Model file for the job. Use its own axes, mm. Round coordinates to 2 decimals unless told otherwise and drop trailing zeros. Loops run counter-clockwise (first coordinate to the right, second up) from the corner with the lowest first, then second, coordinate; pieces in that order, holes last. Notation, with made-up numbers: M 80,-35.5 L 130,-35.5 A19 ccw 130,-30.5 Z; hole C -31,-1 d11. An arc over 180 degrees is marked long. Use a Markdown table: item, result. Add a question column.
Q1. Cut at D-D (x = -63.5). Give the cut face in (y, z).
Q2. Cut at B-B (z = 0). Give the cut face in (x, y).
Q3. Cut at A-A (x = 40.5). Give the cut face in (y, z), plus the area to 3 significant figures.
Q4. Probe line 1 (X direction, y = 1.3, z = 0); line 2 (X direction, y = -1.15, z = -9.5); line 3 (Z direction, x = -63.5, y = -0.45). List the from-to ranges inside material, lowest first. Write a range as from..to.
Q5. Pin check, flat tip, straight feed: pin 1 (2.5 mm diameter, centred on x = -63.5, z = 0, fed in from -Y). Stop position of the tip, or through.
Q6. Cut at C-C (y = 0.15). State how many separate pieces and enclosed holes the cut face has, plus the area to 3 significant figures.
from build123d import *

# Parameters (mm, degrees)
SKETCH1_W           = 152.4
SKETCH1_H           = 63.5
SKETCH1_R           = 1.4605
SKETCH1_W_2         = 16.002
SKETCH1_H_2         = 28.702
BOSS_EXTRUDE1_DEPTH = 2.667
FILLET1_R           = 1.27
FILLET2_R           = 6.35


with BuildPart() as part:
    # Sketch1 → Boss-Extrude1 (new, symmetric)
    with BuildSketch(Plane(origin=(0, 0, 0), x_dir=(1, 0, 0), z_dir=(0, 1, 0))):
        Rectangle(SKETCH1_W, SKETCH1_H)
        with Locations(Location((63.5, 0, 0), (0, 0, 270))):
            Circle(SKETCH1_R, mode=Mode.SUBTRACT)
        with Locations(Location((-63.5, 0, 0), (0, 0, 90))):
            Circle(SKETCH1_R, mode=Mode.SUBTRACT)
        with Locations((-38.1, 0)):
            Rectangle(SKETCH1_W_2, SKETCH1_H_2, mode=Mode.SUBTRACT)
        Rectangle(SKETCH1_W_2, SKETCH1_H_2, mode=Mode.SUBTRACT)
        with Locations((38.1, 0)):
            Rectangle(SKETCH1_W_2, SKETCH1_H_2, mode=Mode.SUBTRACT)
    extrude(amount=BOSS_EXTRUDE1_DEPTH, both=True)

    # Fillet1
    fillet1_edges = [part.edges().sort_by_distance(p)[0] for p in [
        (-30.099, 0, 14.351),
        (-30.099, 0, -14.351),
        (-46.101, 0, -14.351),
        (-46.101, 0, 14.351),
        (8.001, 0, 14.351),
        (8.001, 0, -14.351),
        (-8.001, 0, -14.351),
        (-8.001, 0, 14.351),
        (46.101, 0, 14.351),
        (46.101, 0, -14.351),
        (30.099, 0, -14.351),
        (30.099, 0, 14.351),
    ]]
    fillet(fillet1_edges, radius=FILLET1_R)

    # Fillet2
    fillet2_edges = [part.edges().sort_by_distance(p)[0] for p in [
        (76.2, 0, 31.75),
        (-76.2, 0, 31.75),
        (-76.2, 0, -31.75),
        (76.2, 0, -31.75),
    ]]
    fillet(fillet2_edges, radius=FILLET2_R)


solid = part.part
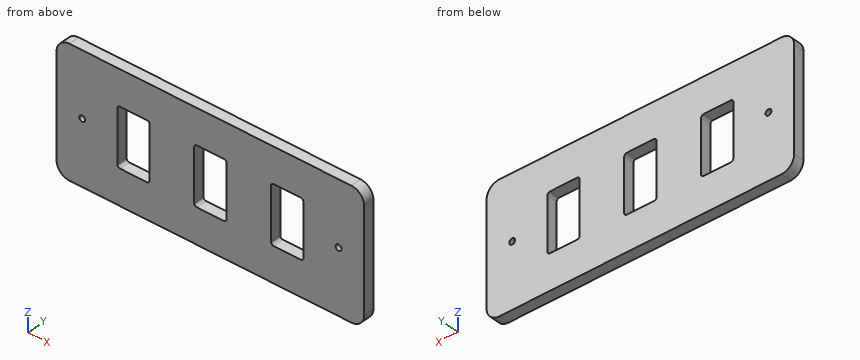
Checked values:
| question | item | result |
|---|---|---|
| 1 | outline | M -2.67,-31.75 L 2.67,-31.75 L 2.67,-1.46 L -2.67,-1.46 Z; M -2.67,1.46 L 2.67,1.46 L 2.67,31.75 L -2.67,31.75 Z |
| 2 | outline | M -76.2,-2.67 L -64.96,-2.67 L -64.96,2.67 L -76.2,2.67 Z; M -62.04,-2.67 L -46.1,-2.67 L -46.1,2.67 L -62.04,2.67 Z; M -30.1,-2.67 L -8,-2.67 L -8,2.67 L -30.1,2.67 Z; M 8,-2.67 L 30.1,-2.67 L 30.1,2.67 L 8,2.67 Z; M 46.1,-2.67 L 62.04,-2.67 L 62.04,2.67 L 46.1,2.67 Z; M 64.96,-2.67 L 76.2,-2.67 L 76.2,2.67 L 64.96,2.67 Z |
| 3 | outline | M -2.67,-31.75 L 2.67,-31.75 L 2.67,-14.35 L -2.67,-14.35 Z; M -2.67,14.35 L 2.67,14.35 L 2.67,31.75 L -2.67,31.75 Z |
| 3 | area | 186 mm^2 |
| 4 | line 1 | x = -76.2..-64.96, -62.04..-46.1, -30.1..-8, 8..30.1, 46.1..62.04, 64.96..76.2 |
| 4 | line 2 | x = -76.2..-46.1, -30.1..-8, 8..30.1, 46.1..76.2 |
| 4 | line 3 | z = -31.75..-1.46, 1.46..31.75 |
| 5 | pin 1 | passes through |
| 6 | separate pieces | 1 |
| 6 | enclosed holes | 5 |
| 6 | area | 8,260 mm^2 |
